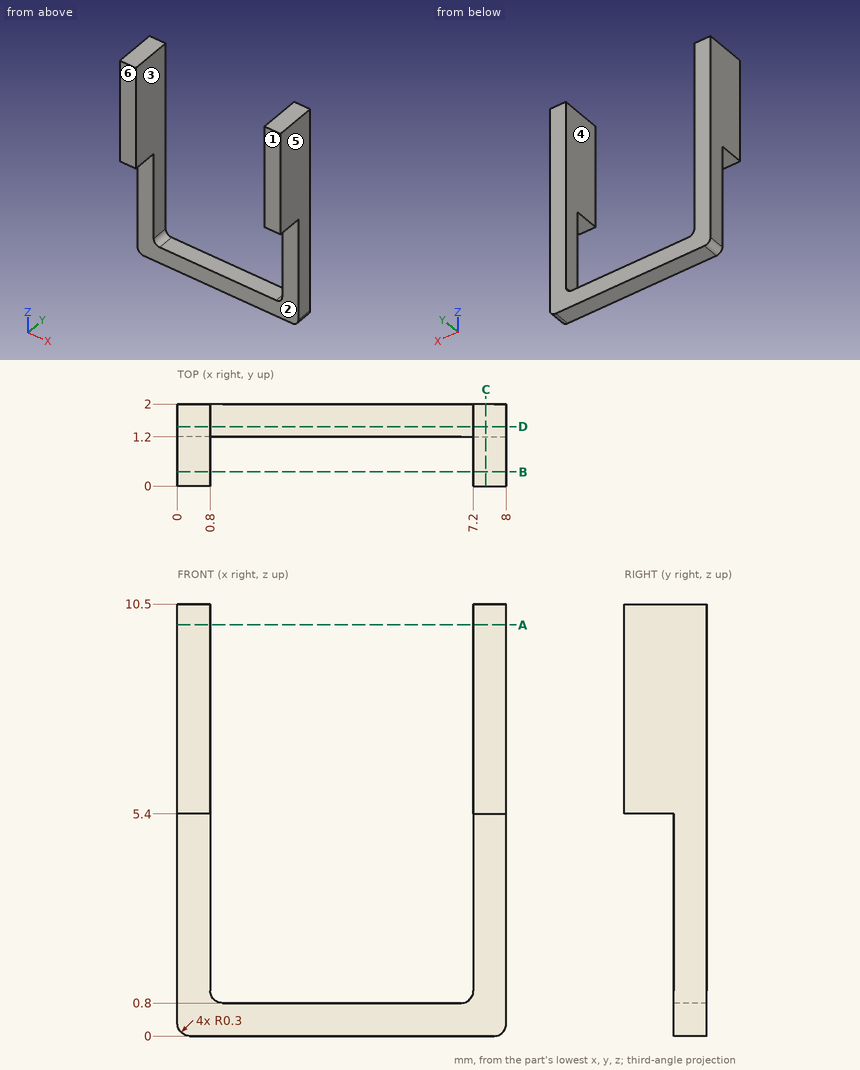
Part print with two shaded views. Sizes in mm from the minimum x, y, z corner. A direction names the side the tool comes from. Coordinates: 2 decimals unless noted, no trailing zeros. Write each loop counter-clockwise with the first axis right and the second up, starting at its lowest first coordinate (ties: lowest second). Pieces come first, ordered by that corner, then holes.
(1) Cut at B-B on y = 0.35. List the corners of the cut face in (x, z).
(2) Drill centre lines: line 1 (X direction, y = 1.65, z = 3.75); line 2 (Z direction, x = 7.25, y = 1); line 3 (Z direction, x = 3, y = 1.7). Where is each one in solid material? Low to high.
(3) Cut at D-D on y = 1.45. List the corners of the cut face in (x, z).
(4) Cut at A-A on z = 10. List the corners of the cut face in (x, y), and give its area (3 significant figures).
(5) Cut at C-C on x = 7.5. List the corners of the cut face in (y, z).
(6) Mould opens along X. For the marked faces 3, 4, 5 and 6 say: pulls with the +X half, pulls with the -X half, needs draft (parallel to the pull), parting line crosses it, or undercut.
(7) Pin check, flat tips, straight feed: pin 1 Ø0.9 at (x, y) = (7.5, 0.5) entering from -Z; pin 2 Ø0.6 at (x, y) = (5.5, 1.5) entering from +Z; pin 3 Ø2 at (x, z) = (6.5, 3.5) entering from -Y. Stop position of each tip, or through.
(8) 3-axis set-ups, long thin cutter, end or side, ignore diameter. For the marked faces 1 and 2: which of +Z, -Z, +X, -X, +Y, -Y reach the whole face in a straight line?
Working result:
1. outline: (0, 5.4) - (0.8, 5.4) - (0.8, 10.5) - (0, 10.5) - close; (7.2, 5.4) - (8, 5.4) - (8, 10.5) - (7.2, 10.5) - close
2. line 1: x = 0 to 0.8, 7.2 to 8
2. line 2: z = 5.4 to 10.5
2. line 3: z = 0 to 0.8
3. outline: (0, 0.3) arc R0.3 ccw to (0.3, 0) - (7.7, 0) arc R0.3 ccw to (8, 0.3) - (8, 10.5) - (7.2, 10.5) - (7.2, 1.1) arc R0.3 cw to (6.9, 0.8) - (1.1, 0.8) arc R0.3 cw to (0.8, 1.1) - (0.8, 10.5) - (0, 10.5) - close
4. outline: (0, 0) - (0.8, 0) - (0.8, 2) - (0, 2) - close; (7.2, 0) - (8, 0) - (8, 2) - (7.2, 2) - close
4. area: 3.20 mm2
5. outline: (0, 5.4) - (1.2, 5.4) - (1.2, 0) - (2, 0) - (2, 10.5) - (0, 10.5) - close
6. face 3: undercut
6. face 4: undercut
6. face 5: pulls with the +X half
6. face 6: needs draft
7. pin 1: stops at z = 5.4
7. pin 2: stops at z = 0.8
7. pin 3: stops at y = 1.2
8. face 1: +Z, -Z, +X, -X, -Y
8. face 2: -Z, +X, -X, -Y
